```python
from build123d import *

# Parameters (mm, degrees)
SKETCH_1_W                  = 80
SKETCH_1_H                  = 60
EXTRUDE_1_DEPTH             = 10
HOLE_WIZARD_M5_1_D          = 4.2
HOLE_WIZARD_8_8_8_8_1_D     = 8.8
HOLE_WIZARD_8_8_8_8_1_DEPTH = 6
HOLE_WIZARD_8_8_8_8_1_TIP   = 2.643786724
HOLE_WIZARD_M6_1_D          = 5
HOLE_WIZARD_M6_1_DEPTH      = 5
HOLE_WIZARD_M6_1_TIP        = 1.502151548


with BuildPart() as part:
    # 스케치1 → 보스-돌출1 (new body)
    with BuildSketch(Plane.XY):
        Rectangle(SKETCH_1_W, SKETCH_1_H)
    extrude(amount=EXTRUDE_1_DEPTH)

    # M5 탭을 위한 탭 드릴1 (through all)
    with Locations(Plane(origin=(-25.5, 0, 10), x_dir=(1, 0, 0), z_dir=(0, 0, 1))):
        with Locations((0, 0), (15.5, -15.5), (31, 0), (15.5, 15.5)):
            Hole(HOLE_WIZARD_M5_1_D / 2)

    # Ø8.8 (8.8) 지름 구멍1
    with Locations(Plane(origin=(-25.5, 0, 10), x_dir=(1, 0, 0), z_dir=(0, 0, 1))):
        with Locations((0, 0), (15.5, 15.5), (31, 0), (15.5, -15.5)):
            Hole(HOLE_WIZARD_8_8_8_8_1_D / 2, depth=HOLE_WIZARD_8_8_8_8_1_DEPTH)
            with Locations((0, 0, -(HOLE_WIZARD_8_8_8_8_1_DEPTH + HOLE_WIZARD_8_8_8_8_1_TIP / 2))):  # 118° drill point
                Cone(0, HOLE_WIZARD_8_8_8_8_1_D / 2, HOLE_WIZARD_8_8_8_8_1_TIP, mode=Mode.SUBTRACT)

    # M6 탭을 위한 탭 드릴1
    with Locations(Plane(origin=(-10, 24, 10), x_dir=(1, 0, 0), z_dir=(0, 0, 1))):
        with Locations((0, 0), (-24, -24), (0, -48), (24, -24)):
            Hole(HOLE_WIZARD_M6_1_D / 2, depth=HOLE_WIZARD_M6_1_DEPTH)
            with Locations((0, 0, -(HOLE_WIZARD_M6_1_DEPTH + HOLE_WIZARD_M6_1_TIP / 2))):  # 118° drill point
                Cone(0, HOLE_WIZARD_M6_1_D / 2, HOLE_WIZARD_M6_1_TIP, mode=Mode.SUBTRACT)


solid = part.part
```
Work out the finished part from the listing and answer in its coordinate system (mm). A direction names the side the tool comes from. Give positions to 0.01 mm unless a question says otherwise; leave off trailing zeros. Loops run counter-clockwise (first coordinate to the right, second up) from the corner with the lowest first, then second, coordinate; pieces in that order, holes last. Notation, with made-up numbers: (74, 47) -> (102, 47) arc R32 ccw to (102, 84) -> close; hole circle Ø1 at (65, 82.25). An arc over 180 degrees is marked (long way). Put each result on its own line as item: value. Start each with the question number.
Item 1: Which of the six approach directions +Z, -Z, +X, -X, +Y, -Y give full straight-line access (tool end or side, diameter ignored) to faces 4 (the face through (-36.31, -0.96, 7.46)), 5 (the face through (-1, 0, 0))?
Item 2: The mould has two halves that part along Y. Classify faces 1 (the face through (-1, -30, 5)), 2 (the face through (9.896, 0.193, 6.958)), 3 (the face through (-1, 0, 10)): released by +Y, released by -Y, zero draft, split by the parting line, or undercut.
Item 3: The part is cut by section C-C (z = 7.5). State how many separate pieces and enclosed holes the cut face has, then the cut area to 3 significant figures.
Item 4: Each of these flat-tipped pins is pushed along its axis until it touches: P1, Ø5.5, axis at x = -25.5, y = 0, coming from the +Z side; P2, Ø8, axis at x = -25.5, y = 0, coming from the +Z side. Where does it stop, or does it pass through?
Item 5: Find the intervals of material crossed by L1, parallel to X at y = 0, z = 8.25; L2, parallel to Y at x = -10, z = 6.85; L3, parallel to Y at x = -25.5, z = 0.65, in increasing order. Write a range as [from, to].
Item 6: The part is cut by section B-B (x = -25.5). Give the vertices of the cut face in (y, z).
Item 7: The part is cut by section A-A (y = -15.5). Give the vertices of the cut face in (x, z).
Answers below:
1. face 4: +Z
1. face 5: -Z, +X, -X, +Y, -Y
2. face 1: released by -Y
2. face 2: undercut
2. face 3: zero draft
3. separate pieces: 1
3. enclosed holes: 8
3. area: 4,480 mm2
4. P1: z = 3.01
4. P2: z = 3.76
5. L1: [-40, -36.5], [-31.5, -29.9], [-21.1, 1.1], [9.9, 11.5], [16.5, 40]
5. L2: [-30, -26.5], [-21.5, -19.9], [-11.1, 11.1], [19.9, 21.5], [26.5, 30]
5. L3: [-30, -2.1], [2.1, 30]
6. outline: (-30, 0) -> (-2.1, 0) -> (-2.1, 2.62) -> (-4.4, 4) -> (-4.4, 10) -> (-30, 10) -> close; (2.1, 0) -> (30, 0) -> (30, 10) -> (4.4, 10) -> (4.4, 4) -> (2.1, 2.62) -> close
7. outline: (-40, 0) -> (-12.1, 0) -> (-12.1, 2.62) -> (-14.4, 4) -> (-14.4, 10) -> (-40, 10) -> close; (-7.9, 0) -> (40, 0) -> (40, 10) -> (-5.6, 10) -> (-5.6, 4) -> (-7.9, 2.62) -> close
